Design review of the part built by this model. Coordinates are the model's own, in mm. A direction names the side the tool comes from. Coordinates: 2 decimals unless noted, no trailing zeros. Write each loop counter-clockwise with the first axis right and the second up, starting at its lowest first coordinate (ties: lowest second). Pieces come first, ordered by that corner, then holes. Notation, with made-up numbers: (-17.75, 51) -> (21.25, 51) arc R11 ccw to (21.25, 65) -> close; hole circle Ø6 at (66.25, 39). An arc over 180 degrees is marked (long way). Write item = value, one per line. Start each with the question number.
```python
from build123d import *

# Parameters (mm, degrees)
SKETCH1_W           = 279.4
SKETCH1_H           = 35.56
BOSS_EXTRUDE1_DEPTH = 9.525
SKETCH2_W           = 12.7
SKETCH2_H           = 9.525
BOSS_EXTRUDE2_DEPTH = 9.525


with BuildPart() as part:
    # Sketch1 → Boss-Extrude1 (new body)
    with BuildSketch(Plane(origin=(0, 0, 0), x_dir=(1, 0, 0), z_dir=(0, 1, 0))):
        Rectangle(SKETCH1_W, SKETCH1_H)
    extrude(amount=BOSS_EXTRUDE1_DEPTH)

    # Sketch2 → Boss-Extrude2 (add)
    with BuildSketch(Plane(origin=(139.7, 0, 0), x_dir=(0, 0, -1), z_dir=(1, 0, 0))):
        with Locations((0, 4.7625)):
            Rectangle(SKETCH2_W, SKETCH2_H)
    boss_extrude2 = extrude(amount=BOSS_EXTRUDE2_DEPTH)

    # Mirror1: Boss-Extrude2 across plane
    add(boss_extrude2.mirror(Plane(origin=(0, 0, 0), x_dir=(0, 0, 1), z_dir=(1, 0, 0))))


solid = part.part
```
(1) For pin 1 Ø3 at (x, y) = (142, 3.5) entering from -Z; pin 2 Ø1.5 at (y, z) = (5.5, 8.5) entering from +X; pin 3 Ø3 at (y, z) = (5.5, 13.5) entering from -X, all flat-tipped, find the tip position at first contact; note any pin that passes through.
(2) For line 1 (X direction, y = 4, z = 15.5), list the stretches that pass through material, from the lowest coordinate up.
(3) Take a section at A-A, the plane y = 4.25. State the section outline as (x, z) points (3 decimals).
(4) For faces 1 (the face through (-144, 5, -6.35)), 2 (the face through (144, 5, 6.35)), 3 (the face through (-139.7, 5, 12)), list the 3-axis set-ups (+Z, -Z, +X, -X, +Y, -Y) from which the entire face can be reached by the end or side of a thin tool; tool diameter is ignored.
(5) Take a section at B-B, the plane z = 9. State the section outline as (x, y) points (3 decimals).
Report:
q1.pin_1 = -6.35
q1.pin_2 = 139.7
q1.pin_3 = -139.7
q2.line_1 = -139.7 to 139.7
q3.outline = (-149.225, -6.35) -> (-139.7, -6.35) -> (-139.7, -17.78) -> (139.7, -17.78) -> (139.7, -6.35) -> (149.225, -6.35) -> (149.225, 6.35) -> (139.7, 6.35) -> (139.7, 17.78) -> (-139.7, 17.78) -> (-139.7, 6.35) -> (-149.225, 6.35) -> close
q4.face_1 = -Z, -X, +Y, -Y
q4.face_2 = +Z, +X, +Y, -Y
q4.face_3 = +Z, -X, +Y, -Y
q5.outline = (-139.7, 0) -> (139.7, 0) -> (139.7, 9.525) -> (-139.7, 9.525) -> close
